The model under review builds one solid part; all positions refer to its coordinate system, in mm. A direction names the side the tool comes from. Round coordinates to 2 decimals unless told otherwise and drop trailing zeros. Order: outer loops, then holes, each group sorted by start corner. A loop starts at its lowest first (then second) coordinate and runs counter-clockwise, first axis right, second up. Notation, with made-up numbers: M -14,57 L 2,57 A25 cw 2,74 Z; hole C -14,-17.75 d10. An arc over 180 degrees is marked long. One line per item, written item: value. Start each with the question number.
from build123d import *

# Parameters (mm, degrees)
BOSS_EXTRUDE1_DEPTH = 25
SKETCH2_R           = 4
CUT_EXTRUDE1_DEPTH  = 31
SKETCH3_R           = 1.6
CUT_EXTRUDE2_DEPTH  = 46
SKETCH4_W           = 10
SKETCH4_H           = 25
CUT_EXTRUDE3_DEPTH  = 26
SKETCH5_R           = 3.5
CUT_EXTRUDE4_DEPTH  = 3


with BuildPart() as part:
    # Sketch1 → Boss-Extrude1 (new body)
    with BuildSketch(Plane(origin=(0, 0, 0), x_dir=(1, 0, 0), z_dir=(0, 1, 0))):
        with BuildLine():
            Line((-14.972375691, 0), (-24.972375691, 0))
            Line((-24.972375691, 0), (-24.972375691, -20))
            Line((-24.972375691, -20), (-4.972375691, -20))
            Line((-4.972375691, -20), (-4.972375691, -45))
            Line((-4.972375691, -45), (5.027624309, -45))
            Line((5.027624309, -45), (5.027624309, -20))
            Line((5.027624309, -20), (25.027624309, -20))
            Line((25.027624309, -20), (25.027624309, 0))
            Line((25.027624309, 0), (15.027624309, 0))
            ThreePointArc((15.027624309, 0), (0.027624309, -15), (-14.972375691, 0))
        make_face()
    extrude(amount=BOSS_EXTRUDE1_DEPTH)

    # Sketch2 → Cut-Extrude1 (cut, through all)
    with BuildSketch(Plane.ZY.offset(4.972375691)):
        with Locations((36, 12.5)):
            Circle(SKETCH2_R)
    extrude(amount=-CUT_EXTRUDE1_DEPTH, mode=Mode.SUBTRACT)

    # Sketch3 → Cut-Extrude2 (cut, through all)
    with BuildSketch(Plane(origin=(0, 0, 0), x_dir=(-1, 0, 0), z_dir=(0, 0, -1))):
        with Locations((-20.027624309, 6.5)):
            Circle(SKETCH3_R)
        with Locations((-20.027624309, 18.5)):
            Circle(SKETCH3_R)
        with Locations((19.972375691, 6.5)):
            Circle(SKETCH3_R)
        with Locations((19.972375691, 18.5)):
            Circle(SKETCH3_R)
    extrude(amount=-CUT_EXTRUDE2_DEPTH, mode=Mode.SUBTRACT)

    # Sketch4 → Cut-Extrude3 (cut, through all)
    with BuildSketch(Plane(origin=(0, 25, 0), x_dir=(1, 0, 0), z_dir=(0, 1, 0))):
        with Locations((0.027624309, -32.5)):
            Rectangle(SKETCH4_W, SKETCH4_H)
    extrude(amount=-CUT_EXTRUDE3_DEPTH, mode=Mode.SUBTRACT)

    # Sketch5 → Cut-Extrude4 (cut)
    with BuildSketch(Plane.XY.offset(20)):
        with Locations((20.027624309, 18.5)):
            Circle(SKETCH5_R)
        with Locations((20.027624309, 6.5)):
            Circle(SKETCH5_R)
        with Locations((-19.972375691, 6.5)):
            Circle(SKETCH5_R)
        with Locations((-19.972375691, 18.5)):
            Circle(SKETCH5_R)
    extrude(amount=-CUT_EXTRUDE4_DEPTH, mode=Mode.SUBTRACT)


solid = part.part
Item 1: The part is to be moulded in two halves that separate along Y. For faces 1 (the flat face through (-18, 18, 17)), 2 (the flat face through (0, 25, 17)), 3 (the flat face through (-20, 12, 0)), say which applies: pulls with the +Y half, pulls with the -Y half, needs draft (parallel to the pull), parting line crosses it, or undercut.
Item 2: Consider section C-C, the plane z = 14.5. Give the boundary of the cut face in (x, y).
Item 3: Consider section D-D, the plane y = 5.5. Give the boundary of the cut face in (x, z), then the cut area to 3 significant figures.
Item 4: Clearance check with flat-ended pins moving along their axes: P1, Ø11, axis at x = 20.03, y = 6.5, coming from the +Z side; P2, Ø4, axis at x = 7.5, y = 9.5, coming from the -Z side; P3, Ø5.5, axis at x = -20, y = 6.5, coming from the +Z side. State where each tip first meets the part, or that it passes through.
Item 5: Machinability: for faces 4 (the cylindrical face through (19.29, 5.08, 8.38)), 5 (the flat face through (-18, 6, 17)), which of the approach directions +Z, -Z, +X, -X, +Y, -Y give a long, thin tool a straight path to every point of the face, cutting with its end or side? Answer none if there is none.
Item 6: Consider section A-A, the plane z = 3.25. Give the boundary of the cut face in (x, y), then the cut area to 3 significant figures.
Item 7: Consider section B-B, the plane y = 18.5. Give the boundary of the cut face in (x, z), then the cut area to 3 significant figures.
Item 8: Wall thickness on L1, parallel to Y at x = -20, z = 5.5; L2, parallel to X at y = 19.75, z = 3.25; L3, parallel to Y at x = 21, z = 12.25: over which ranges is each line inside the solid? List them lowest first.
Computed:
1. face 1: undercut
1. face 2: pulls with the +Y half
1. face 3: needs draft
2. outline: M -24.97,0 L -3.81,0 L -3.81,25 L -24.97,25 Z; M 3.87,0 L 25.03,0 L 25.03,25 L 3.87,25 Z; hole C -19.97,6.5 d3.2; hole C -19.97,18.5 d3.2; hole C 20.03,6.5 d3.2; hole C 20.03,18.5 d3.2
3. outline: M -24.97,0 L -21.22,0 L -21.22,17 L -23.33,17 L -23.33,20 L -24.97,20 Z; M -18.72,0 L -14.97,0 A15 cw 15.03,0 L 18.78,0 L 18.78,17 L 16.67,17 L 16.67,20 L -16.62,20 L -16.62,17 L -18.72,17 Z; M 21.28,0 L 25.03,0 L 25.03,20 L 23.38,20 L 23.38,17 L 21.28,17 Z
3. area: 521 mm^2
4. P1: stops at z = 20
4. P2: stops at z = 11.63
4. P3: stops at z = 17
5. face 4: +Z, -Z
5. face 5: +Z
6. outline: M -24.97,0 L -14.62,0 L -14.62,25 L -24.97,25 Z; M 14.67,0 L 25.03,0 L 25.03,25 L 14.67,25 Z; hole C -19.97,6.5 d3.2; hole C -19.97,18.5 d3.2; hole C 20.03,6.5 d3.2; hole C 20.03,18.5 d3.2
6. area: 486 mm^2
7. outline: M -24.97,0 L -21.57,0 L -21.57,17 L -23.47,17 L -23.47,20 L -24.97,20 Z; M -18.37,0 L -14.97,0 A15 cw 15.03,0 L 18.43,0 L 18.43,17 L 16.53,17 L 16.53,20 L -16.47,20 L -16.47,17 L -18.37,17 Z; M 21.63,0 L 25.03,0 L 25.03,20 L 23.53,20 L 23.53,17 L 21.63,17 Z
7. area: 496 mm^2
8. L1: y = 0 to 4.9, 8.1 to 16.9, 20.1 to 25
8. L2: x = -24.97 to -20.97, -18.97 to -14.62, 14.67 to 19.03, 21.03 to 25.03
8. L3: y = 0 to 5.23, 7.77 to 17.23, 19.77 to 25
